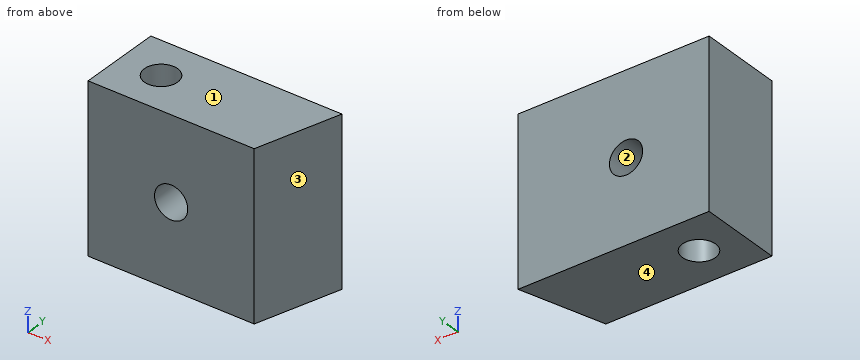
```python
from build123d import *

# Parameters (mm, degrees)
F0_W     = 20
F0_H     = 10
F1_DEPTH = 10
F2_DEPTH = 10
F3_DEPTH = 20
F4_R     = 2
F5_DEPTH = 25
F6_R     = 2
F7_DEPTH = 25


with BuildPart() as f1:
    # F0 (on Top) → F1 (new body)
    with BuildSketch(Plane.XY):
        with Locations((10, 5)):
            Rectangle(F0_W, F0_H)
    extrude(amount=F1_DEPTH)

    # F0 (on Top) → F2 (join)
    with BuildSketch(Plane.XY):
        with Locations((10, 5)):
            Rectangle(F0_W, F0_H)
        Polygon((20, 10), (20, 0), (23, 10), align=None)
    extrude(amount=F2_DEPTH)

    # F0 (on Top) → F3 (join)
    with BuildSketch(Plane.XY):
        with Locations((10, 5)):
            Rectangle(F0_W, F0_H)
        Polygon((20, 10), (20, 0), (23, 10), align=None)
    extrude(amount=F3_DEPTH)

    # F4 (on face) → F5 (cut)
    with BuildSketch(Plane(origin=(0, 10, 0), x_dir=(-1, 0, 0), z_dir=(0, 1, 0))):
        with Locations((-10, 10)):
            Circle(F4_R)
    extrude(amount=-F5_DEPTH, mode=Mode.SUBTRACT)

    # F6 (on face) → F7 (cut)
    with BuildSketch(Plane.XY.offset(20)):
        with Locations((5, 5)):
            Circle(F6_R)
    extrude(amount=-F7_DEPTH, mode=Mode.SUBTRACT)


solid = f1.part
```
Check sheet for the modelled part. Datum: model origin and axes. Units: mm. Face numbers are marked on the shaded views. Round coordinates to 2 decimals unless told otherwise and drop trailing zeros. Loops run counter-clockwise (first coordinate to the right, second up) from the corner with the lowest first, then second, coordinate; pieces in that order, holes last. Notation, with made-up numbers: (46.5, 0) -> (82.5, 0) arc R23 ccw to (82.5, 22) -> close; hole circle Ø5 at (11, 6). An arc over 180 degrees is marked (long way). Answer in a Markdown table with one row per item.
Q1. Release check for a two-part mould opening along Z. For the marked faces 1, 2, 3 and 4 record: released by +Z, released by -Z, zero draft, split by the parting line, or undercut.
Data:
| item | result |
|---|---|
| face 1 | released by +Z |
| face 2 | undercut |
| face 3 | zero draft |
| face 4 | released by -Z |
Q2. Sectioned sample at B-B on z = 10. Enter the section's corners in (x, y), then the cut area to 3 significant figures.
Data:
| item | result |
|---|---|
| outline | (0, 0) -> (8, 0) -> (8, 10) -> (0, 10) -> close; (12, 0) -> (20, 0) -> (23, 10) -> (12, 10) -> close; hole circle Ø4 at (5, 5) |
| area | 162 mm^2 |
Q3. Thickness scan on L1, parallel to Z at x = 10, y = 0.5; L2, parallel to X at y = 4.75, z = 9.5 (1 decimal); L3, parallel to Y at x = 5, z = 2.25. Record the ranges inside material, lowest first.
Data:
| item | result |
|---|---|
| L1 | z = 0 to 8, 12 to 20 |
| L2 | x = 0 to 3, 7 to 8.1, 11.9 to 21.4 |
| L3 | y = 0 to 3, 7 to 10 |
Q4. Sectioned sample at C-C on y = 5. Enter the section's corners in (x, z).
Data:
| item | result |
|---|---|
| outline | (0, 0) -> (3, 0) -> (3, 20) -> (0, 20) -> close; (7, 0) -> (21.5, 0) -> (21.5, 20) -> (7, 20) -> close; hole circle Ø4 at (10, 10) |
Q5. Go/stop test with flat-tipped pins: P1, Ø1.5, axis at y = 2.5, z = 10, coming from the +X side (3 decimals); P2, Ø6, axis at y = 6, z = 8.5, coming from the +X side; P3, Ø6, axis at y = 3.5, z = 11.5, coming from the +X side. Record where each tip stops, or that it passes through.
Data:
| item | result |
|---|---|
| P1 | stops at x = 20.975 |
| P2 | stops at x = 22.7 |
| P3 | stops at x = 21.95 |
Q6. Sectioned sample at A-A on x = 5. Enter the section's corners in (y, z).
Data:
| item | result |
|---|---|
| outline | (0, 0) -> (3, 0) -> (3, 20) -> (0, 20) -> close; (7, 0) -> (10, 0) -> (10, 20) -> (7, 20) -> close |
Q7. Sectioned sample at D-D on x = 10. Enter the section's corners in (y, z).
Data:
| item | result |
|---|---|
| outline | (0, 0) -> (10, 0) -> (10, 8) -> (0, 8) -> close; (0, 12) -> (10, 12) -> (10, 20) -> (0, 20) -> close |
